Autodesk Inventor part; units mm, degrees
ref_plane "YZ Plane" through (0, 0, 0) normal (1, 0, 0) x (0, 1, 0)
ref_plane "XZ Plane" through (0, 0, 0) normal (0, 1, 0) x (-1, 0, 0)
ref_plane "XY Plane" through (0, 0, 0) normal (0, 0, 1) x (1, 0, 0)
sketch "스케치1" plane through (0, 0, 0) normal (1, 0, 0) x (0, 1, 0)
  line L0 (0, 0) -> (6.5, 0)
  line L1 (6.5, 0) -> (6.5, 20)
  line L2 (6.5, 20) -> (0, 20)
  line L3 (0, 20) -> (0, 0)
  line L4 (0, 20) -> (8, 20)
  line L5 (8, 20) -> (8, 50)
  line L6 (8, 50) -> (0, 50)
  line L7 (0, 50) -> (0, 20)
  line L8 (0, 50) -> (13.5, 50)
  line L9 (13.5, 50) -> (13.5, 70)
  line L10 (13.5, 70) -> (0, 70)
  line L11 (0, 70) -> (0, 50)
  line L12 (0, 70) -> (8, 70)
  line L13 (8, 70) -> (8, 95)
  line L14 (8, 95) -> (0, 95)
  line L15 (0, 95) -> (0, 70)
  dimension "d0" = 13
  dimension "d1" = 16
  dimension "d2" = 27
  dimension "d3" = 16
  dimension "d4" = 20
  dimension "d5" = 30
  dimension "d6" = 20
  dimension "d7" = 25
revolve "회전1" add sketch "스케치1" angle 360 about axis through (0, 0, 50) along (0, 0, -1)
sketch "스케치2" plane through (0, 0, 0) normal (0, 0, -1) x (-1, 0, 0)
  line L0 (0, 7.0711) -> (7.0711, 0)
  line L1 (7.0711, 0) -> (0, -7.0711)
  line L2 (0, -7.0711) -> (-7.0711, 0)
  line L3 (-7.0711, 0) -> (0, 7.0711)
  circle A0 centre (0, 0) radius 9.2868
  dimension "d9" = 10
extrude "돌출1" cut sketch "스케치2" against normal blind 13
chamfer "모따기1" distance 1 angle 45 5 edges at (-0.2997, 6.4931, 0) (-6.5, 0, 0) (6.5, 0, 0) (0.2997, 6.4931, 0) (0, -6.5, 0)
sketch "스케치3" plane through (0, 0, 70) normal (0, 0, 1) x (1, 0, 0)
  circle A0 centre (0, 0) radius 13.5
  line L0 (-10.0623, 9) -> (-10.0623, -9)
  line L1 (-10.0623, 9) -> (-13.5, 9)
  line L2 (-13.5, 9) -> (-13.5, -9)
  line L3 (-13.5, -9) -> (-10.0623, -9)
  dimension "d15" = 18
extrude "돌출2" cut sketch "스케치3" against normal blind 7 contours L0 A0 | A0 L2 L1 | L3 L2 A0 picked at (-11.0757, -1.0838)
mirror "미러1" about plane through (0, 0, 0) normal (1, 0, 0) of "돌출2"
sketch "스케치4" plane through (0, 0, 0) normal (1, 0, 0) x (0, 1, 0)
  line L0 (8, 92.35) -> (7.6, 92.35)
  line L1 (7.6, 92.35) -> (7.6, 93.5)
  line L2 (7.6, 93.5) -> (8, 93.5)
  line L3 (8, 93.5) -> (8, 92.35)
  line L4 (8, 95) -> (8, 70)
  line L5 (0, -19) -> (0, 114)
  point P0 (0, 0)
  dimension "d19" = 1.15
  dimension "d20" = 1.5
  dimension "d21" = 0.4
revolve "회전2" cut sketch "스케치4" angle 360 about axis through (0, 0, -10) along (0, 0, 1)
chamfer "모따기2" distance 1 angle 45 1 edges at (0, -8, 95)
properties part number "3강"
Source: CAD feature listing. Evaluate the final solid. Frame: model axes, mm. A direction names the side the tool comes from. Give positions to 0.01 mm unless a question says otherwise; leave off trailing zeros. Order: outer loops, then holes, each group sorted by start corner. A loop starts at its lowest first (then second) coordinate and runs counter-clockwise, first axis right, second up. Notation, with made-up numbers: (-35.75, 77) -> (-4.75, 77) arc R14 ccw to (-4.75, 83) -> close; hole circle Ø7 at (74.25, 32). An arc over 180 degrees is marked (long way). Use a Markdown table: item, result.
1) Contact query for flat-ended pins moving along their axis: P1, Ø12, axis at x = 5, z = 74, coming from the -Y side; P2, Ø3, axis at x = 12.5, y = -3, coming from the +Z side; P3, Ø1, axis at x = 8, y = -2, coming from the +Z side. Output: stop coordinate, or through.
Answer list:
| item | result |
|---|---|
| P1 | y = -13.49 |
| P2 | z = 63 |
| P3 | z = 94.25 |
2) Section query A-A, the plane z = 47.5. Return the cut outline in (x, y).
Answer list:
| item | result |
|---|---|
| outline | circle Ø16 at (0, 0) |
3) Ray query, line 1 along Z through (x, y) = (8.25, -7.5); line 2 along X through (y, z) = (-0.75, 16); line 3 along Z through (x, y) = (-6.5, -0.75). Return the intervals inside material, ascending. Write a range as [from, to].
Answer list:
| item | result |
|---|---|
| line 1 | [50, 70] |
| line 2 | [-6.46, 6.46] |
| line 3 | [20, 95] |
4) Reachability of faces 1 (the flat face through (-3.58, -3.49, 6.41)), 2 (the flat face through (-10.062, 0, 67)), 3 (the flat face through (4, 4, 13)), 4 (the flat face through (11, 0, 63)), 5 (the flat face through (7, 0, 20)) from +Z, -Z, +X, -X, +Y, -Y: full face, straight path, thin tool, end or side. Return the list, or none.
Answer list:
| item | result |
|---|---|
| face 1 | -Z, -X, -Y |
| face 2 | +Z, -X, +Y, -Y |
| face 3 | -Z, +X, +Y |
| face 4 | +Z, +X, +Y, -Y |
| face 5 | -Z |
5) Section query B-B, the plane z = 60. Return the cut outline in (x, y).
Answer list:
| item | result |
|---|---|
| outline | circle Ø27 at (0, 0) |
6) Mould query, pull axis Z, two halves, no side actions, for faces 6 (the flat face through (-4, 4, 13)), 7 (the flat face through (10.062, 0, 67)), 8 (the flat face through (-9, 0, 70)), 9 (the cylindrical face through (-0.334, -7.593, 92.933)). Classes: +Z half, -Z half, draft (parallel to the pull), parting line (faces both ways), or undercut.
Answer list:
| item | result |
|---|---|
| face 6 | -Z half |
| face 7 | draft |
| face 8 | +Z half |
| face 9 | undercut |
